Design review of the part built by this model. Coordinates are the model's own, in mm. Face numbers are marked on the shaded views. A direction names the side the tool comes from. Coordinates: 2 decimals unless noted, no trailing zeros. Write each loop counter-clockwise with the first axis right and the second up, starting at its lowest first coordinate (ties: lowest second). Pieces come first, ordered by that corner, then holes. Notation, with made-up numbers: M -7.5,11.25 L 17.5,11.25 A23 ccw 17.5,42.25 Z; hole C -19,-9 d2. An arc over 180 degrees is marked long. Write item = value, one per line.
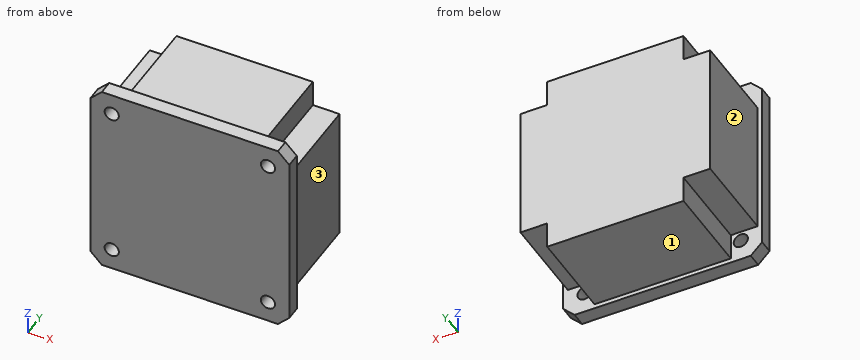
```python
from build123d import *

# Parameters (mm, degrees)
SKETCH2_W                                  = 44.45
SKETCH2_H                                  = 44.45
BOSS_EXTRUDE1_DEPTH                        = 3.175
CHAMFER1_SIZE                              = 2.54
SKETCH3_R                                  = 1.5875
CUT_EXTRUDE1_DEPTH                         = 4.175
MIRROR2_COPY_1_SKETCH_R                    = 1.5875
MIRROR2_COPY_1_DEPTH                       = 4.175
SKETCH4_W                                  = 42.418
SKETCH4_H                                  = 42.418
BOSS_EXTRUDE2_DEPTH                        = 20.1422
SKETCH5_W                                  = 5.969
SKETCH5_H                                  = 5.9817
CUT_EXTRUDE2_DEPTH                         = 20.1422
MIRROR3_AT_THE_SECOND_PLANE_COPY_1_SKETC_W = 5.969
MIRROR3_AT_THE_SECOND_PLANE_COPY_1_SKETC_H = 5.9817
MIRROR3_AT_THE_SECOND_PLANE_COPY_1_DEPTH   = 20.1422


with BuildPart() as part:
    # Sketch2 → Boss-Extrude1 (new body)
    with BuildSketch(Plane(origin=(0, 0, 0), x_dir=(1, 0, 0), z_dir=(0, 1, 0))):
        Rectangle(SKETCH2_W, SKETCH2_H)
    extrude(amount=BOSS_EXTRUDE1_DEPTH)

    # Chamfer1
    chamfer1_edges = [part.edges().sort_by_distance(p)[0] for p in [
        (22.225, 1.5875, 22.225),
        (-22.225, 1.5875, 22.225),
        (-22.225, 1.5875, -22.225),
        (22.225, 1.5875, -22.225),
    ]]
    chamfer(chamfer1_edges, length=CHAMFER1_SIZE)

    # Sketch3 → Cut-Extrude1 (cut, through all)
    with BuildSketch(Plane(origin=(0, 3.175, 0), x_dir=(1, 0, 0), z_dir=(0, 1, 0))):
        with Locations((-17.4625, 17.4625)):
            Circle(SKETCH3_R)
    cut_extrude1 = extrude(amount=-CUT_EXTRUDE1_DEPTH, mode=Mode.SUBTRACT)

    # Mirror1: Cut-Extrude1 across plane
    add(cut_extrude1.mirror(Plane(origin=(0, 0, 0), x_dir=(0, 0, 1), z_dir=(1, 0, 0))), mode=Mode.SUBTRACT)

    # Mirror2: Cut-Extrude1 across plane
    add(cut_extrude1.mirror(Plane.XY), mode=Mode.SUBTRACT)

    # Mirror2 copy 1 sketch → Mirror2 copy 1 (cut, through all)
    with BuildSketch(Plane(origin=(0, 3.175, 0), x_dir=(-1, 0, 0), z_dir=(0, 1, 0))):
        with Locations((-17.4625, 17.4625)):
            Circle(MIRROR2_COPY_1_SKETCH_R)
    extrude(amount=-MIRROR2_COPY_1_DEPTH, mode=Mode.SUBTRACT)

    # Sketch4 → Boss-Extrude2 (add)
    with BuildSketch(Plane(origin=(0, 3.175, 0), x_dir=(1, 0, 0), z_dir=(0, 1, 0))):
        Rectangle(SKETCH4_W, SKETCH4_H)
    extrude(amount=BOSS_EXTRUDE2_DEPTH)

    # Sketch5 → Cut-Extrude2 (cut)
    with BuildSketch(Plane(origin=(0, 23.3172, 0), x_dir=(1, 0, 0), z_dir=(0, 1, 0))):
        with Locations((-18.2245, 18.21815)):
            Rectangle(SKETCH5_W, SKETCH5_H)
    cut_extrude2 = extrude(amount=-CUT_EXTRUDE2_DEPTH, mode=Mode.SUBTRACT)

    # Mirror3: Cut-Extrude2 across plane
    add(cut_extrude2.mirror(Plane(origin=(0, 0, 0), x_dir=(0, 0, 1), z_dir=(1, 0, 0))), mode=Mode.SUBTRACT)

    # Mirror3 at the second plane: Cut-Extrude2 across plane
    add(cut_extrude2.mirror(Plane.XY), mode=Mode.SUBTRACT)

    # Mirror3 at the second plane copy 1 sketc → Mirror3 at the second plane copy 1 (cut)
    with BuildSketch(Plane(origin=(0, 23.3172, 0), x_dir=(-1, 0, 0), z_dir=(0, 1, 0))):
        with Locations((-18.2245, 18.21815)):
            Rectangle(MIRROR3_AT_THE_SECOND_PLANE_COPY_1_SKETC_W, MIRROR3_AT_THE_SECOND_PLANE_COPY_1_SKETC_H)
    extrude(amount=-MIRROR3_AT_THE_SECOND_PLANE_COPY_1_DEPTH, mode=Mode.SUBTRACT)


solid = part.part
```
Q1. Machinability: for the marked faces 1, 2 and 3, which of the approach directions +Z, -Z, +X, -X, +Y, -Y give a long, thin tool a straight path to every point of the face, cutting with its end or side? Answer none if there is none.
Check result:
face_1 = -Z, +X, -X, +Y
face_2 = +Z, -Z, -X, +Y
face_3 = +Z, -Z, +X, +Y
Q2. Consider section D-D, the plane x = -17.5. State the section outline as (y, z) points (3 decimals).
Check result:
outline = M 0,-22.225 L 3.175,-22.225 L 3.175,-19.05 L 0,-19.05 Z; M 0,-15.875 L 3.175,-15.875 L 3.175,-15.227 L 23.317,-15.227 L 23.317,15.227 L 3.175,15.227 L 3.175,15.875 L 0,15.875 Z; M 0,19.05 L 3.175,19.05 L 3.175,22.225 L 0,22.225 Z
Q3. For P1, Ø1.5, axis at y = 8.5, z = 14.5, coming from the -X side; P2, Ø1.8, axis at y = 18, z = 18.5, coming from the +X side; P3, Ø3.5, axis at x = -17.46, z = -17.46, coming from the -Y side; P4, Ø5, axis at x = 18, y = 11, coming from the +Z side, all flat-tipped, find the tip position at first contact; note any pin that passes through.
Check result:
P1 = -21.21
P2 = 15.24
P3 = 0
P4 = 15.23
Q4. Wall thickness on line 1 (Z direction, x = -13, y = 19.25); line 2 (X direction, y = 17.75, z = 19.5): over which ranges is each line inside the solid? List them lowest first.
Check result:
line_1 = -21.21 to 21.21
line_2 = -15.24 to 15.24
Q5. Consider section B-B, the plane z = -9. State the section outline as (x, y) points (3 decimals), and give its area (3 significant figures).
Check result:
outline = M -22.225,0 L 22.225,0 L 22.225,3.175 L 21.209,3.175 L 21.209,23.317 L -21.209,23.317 L -21.209,3.175 L -22.225,3.175 Z
area = 996 mm²
Q6. Consider section A-A, the plane x = -11. State the section outline as (y, z) points (3 decimals), and give its area (3 significant figures).
Check result:
outline = M 0,-22.225 L 3.175,-22.225 L 3.175,-21.209 L 23.317,-21.209 L 23.317,21.209 L 3.175,21.209 L 3.175,22.225 L 0,22.225 Z
area = 996 mm²
Q7. Consider section C-C, the plane y = 9.75. State the section outline as (x, z) points.
Check result:
outline = M -21.21,-15.23 L -15.24,-15.23 L -15.24,-21.21 L 15.24,-21.21 L 15.24,-15.23 L 21.21,-15.23 L 21.21,15.23 L 15.24,15.23 L 15.24,21.21 L -15.24,21.21 L -15.24,15.23 L -21.21,15.23 Z
